Part model, mm, in its own coordinate system. Face numbers are marked on the shaded views. Give positions to 0.01 mm unless a question says otherwise; leave off trailing zeros. Write each loop counter-clockwise with the first axis right and the second up, starting at its lowest first coordinate (ties: lowest second). Pieces come first, ordered by that corner, then holes. Notation, with made-up numbers: M 7,-34.75 L 36,-34.75 A20 ccw 36,-21.75 Z; hole C 4.25,0.25 d3. An arc over 180 degrees is marked long. Use CSV: the item, a comma, the result in double quotes. Start each with the question number.
Item 1: Drill centre lines: line 1 (Y direction, x = 50.8, z = 26); line 2 (Y direction, x = 50, z = 9); line 3 (Z direction, x = 25.5, y = -4.5). Where is each one in solid material? Low to high. Write a range as [from, to].
Item 2: Mould opens along X. For the marked faces 1 and 2 say: released by +X, released by -X, zero draft, split by the parting line, or undercut.
Item 3: Cut at D-D (x = 73). List the corners of the cut face in (y, z), then the cut area to 3 significant figures.
Item 4: Pin check, flat tips, straight feed: pin 1 (4 mm diameter, centred on y = -2.5, z = 32.5, fed in from -X); pin 2 (8 mm diameter, centred on y = -12, z = 37.5, fed in from -X); pin 3 (3 mm diameter, centred on y = -21.5, z = 17, fed in from +X); pin 4 (7.5 mm diameter, centred on x = 50.8, y = -9.652, fed in from +Z). Stop position of each tip, or through.
Item 5: Cut at A-A (x = 92.5). List the corners of the cut face in (y, z).
Item 6: Cut at B-B (y = -8.5). List the corners of the cut face in (x, z), then the cut area to 3 significant figures.
Item 7: Cut at C-C (z = 5). List the corners of the cut face in (x, y).
from build123d import *

# Parameters (mm, degrees)
F1_DEPTH = 6.35
F2_R     = 4.7625
F3_DEPTH = 63.5
F4_R     = 12.7
F5_DEPTH = 63.5


with BuildPart() as f1:
    # F0 (on Top) → F1 (new body)
    with BuildSketch(Plane.XY):
        with BuildLine():
            Line((0, 7.874), (0, 0))
            Line((0, 0), (15.748, 0))
            ThreePointArc((15.748, 0), (25.4, -9.652), (15.748, -19.304))
            Line((15.748, -19.304), (0, -19.304))
            Line((0, -19.304), (0, -27.178))
            ThreePointArc((0, -27.178), (0.446369, -28.255631), (1.524, -28.702))
            Line((1.524, -28.702), (100.076, -28.702))
            ThreePointArc((100.076, -28.702), (101.153631, -28.255631), (101.6, -27.178))
            Line((101.6, -27.178), (101.6, -19.304))
            Line((101.6, -19.304), (85.852, -19.304))
            ThreePointArc((85.852, -19.304), (76.2, -9.652), (85.852, 0))
            Line((85.852, 0), (101.6, 0))
            Line((101.6, 0), (101.6, 7.874))
            ThreePointArc((101.6, 7.874), (101.153631, 8.951631), (100.076, 9.398))
            Line((100.076, 9.398), (1.524, 9.398))
            ThreePointArc((1.524, 9.398), (0.446369, 8.951631), (0, 7.874))
        make_face()
    extrude(amount=-F1_DEPTH)

    # F2 (on face) → F3 (join)
    with BuildSketch(Plane.XY):
        with BuildLine():
            ThreePointArc((50.8, -28.702), (64.270384, -23.122384), (69.85, -9.652))
            ThreePointArc((69.85, -9.652), (64.270384, 3.818384), (50.8, 9.398))
            ThreePointArc((50.8, 9.398), (31.75, -9.652), (50.8, -28.702))
        make_face()
        with Locations((50.8, -9.652)):
            Circle(F2_R, mode=Mode.SUBTRACT)
    extrude(amount=F3_DEPTH)

    # F4 (on face) → F5 (cut)
    with BuildSketch(Plane(origin=(0, 0, -6.35), x_dir=(1, 0, 0), z_dir=(0, 0, -1))):
        with Locations((50.8, 9.652)):
            Circle(F4_R)
    extrude(amount=-F5_DEPTH, mode=Mode.SUBTRACT)


solid = f1.part
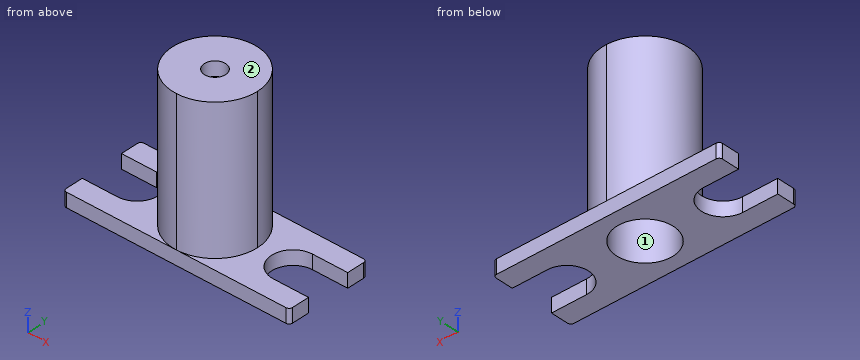
Worked answers:
1,line 1,"y = [-28.7, -22.35], [3.05, 9.4]"
1,line 2,"y = [-28.69, -22.33], [3.02, 9.38]"
1,line 3,"z = [-6.35, 0]"
2,face 1,"undercut"
2,face 2,"zero draft"
3,outline,"M -28.7,-6.35 L 9.4,-6.35 L 9.4,0 L -28.7,0 Z"
3,area,"242 mm^2"
4,pin 1,"stops at x = 32.46"
4,pin 2,"stops at x = 31.75"
4,pin 3,"stops at x = 66.79"
4,pin 4,"passes through"
5,outline,"M -28.7,-6.35 L -19.3,-6.35 L -19.3,0 L -28.7,0 Z; M 0,-6.35 L 9.4,-6.35 L 9.4,0 L 0,0 Z"
6,outline,"M 25.33,-6.35 L 38.15,-6.35 L 38.15,57.15 L 46.18,57.15 L 46.18,63.5 L 31.78,63.5 L 31.78,0 L 25.33,0 Z; M 55.42,57.15 L 63.45,57.15 L 63.45,-6.35 L 76.27,-6.35 L 76.27,0 L 69.82,0 L 69.82,63.5 L 55.42,63.5 Z"
6,area,"1,070 mm^2"
7,outline,"M 50.8,-28.7 A19.05 ccw 69.85,-9.65 A19.05 ccw long Z; hole C 50.8,-9.65 d25.4"
